from build123d import *

# Parameters (mm, degrees)
SKETCH_1_W      = 303
SKETCH_1_H      = 10
SKETCH_1_R      = 2.025
EXTRUDE_1_DEPTH = 4
FILLET_1_R      = 2


with BuildPart() as part:
    # 草图1 → 凸台-拉伸1 (new body)
    with BuildSketch(Plane.XY):
        Rectangle(SKETCH_1_W, SKETCH_1_H)
        with Locations((-112, 0)):
            Circle(SKETCH_1_R, mode=Mode.SUBTRACT)
        with Locations((-98, 0)):
            Circle(SKETCH_1_R, mode=Mode.SUBTRACT)
        with Locations((-84, 0)):
            Circle(SKETCH_1_R, mode=Mode.SUBTRACT)
        with Locations((-70, 0)):
            Circle(SKETCH_1_R, mode=Mode.SUBTRACT)
        with Locations((-56, 0)):
            Circle(SKETCH_1_R, mode=Mode.SUBTRACT)
        with Locations((-42, 0)):
            Circle(SKETCH_1_R, mode=Mode.SUBTRACT)
        with Locations((-28, 0)):
            Circle(SKETCH_1_R, mode=Mode.SUBTRACT)
        with Locations((-14, 0)):
            Circle(SKETCH_1_R, mode=Mode.SUBTRACT)
        Circle(SKETCH_1_R, mode=Mode.SUBTRACT)
        with Locations((14, 0)):
            Circle(SKETCH_1_R, mode=Mode.SUBTRACT)
        with Locations((28, 0)):
            Circle(SKETCH_1_R, mode=Mode.SUBTRACT)
        with Locations((42, 0)):
            Circle(SKETCH_1_R, mode=Mode.SUBTRACT)
        with Locations((56, 0)):
            Circle(SKETCH_1_R, mode=Mode.SUBTRACT)
        with Locations((70, 0)):
            Circle(SKETCH_1_R, mode=Mode.SUBTRACT)
        with Locations((84, 0)):
            Circle(SKETCH_1_R, mode=Mode.SUBTRACT)
        with Locations((98, 0)):
            Circle(SKETCH_1_R, mode=Mode.SUBTRACT)
        with Locations((112, 0)):
            Circle(SKETCH_1_R, mode=Mode.SUBTRACT)
        with Locations((-144.5, 0)):
            Circle(SKETCH_1_R, mode=Mode.SUBTRACT)
        with Locations((-130.5, 0)):
            Circle(SKETCH_1_R, mode=Mode.SUBTRACT)
        with Locations((130.5, 0)):
            Circle(SKETCH_1_R, mode=Mode.SUBTRACT)
        with Locations((144.5, 0)):
            Circle(SKETCH_1_R, mode=Mode.SUBTRACT)
    extrude(amount=EXTRUDE_1_DEPTH)

    # 圆角1
    fillet_1_edges = [part.edges().sort_by_distance(p)[0] for p in [
        (151.5, -5, 2),
        (-151.5, -5, 2),
        (-151.5, 5, 2),
        (151.5, 5, 2),
    ]]
    fillet(fillet_1_edges, radius=FILLET_1_R)


solid = part.part
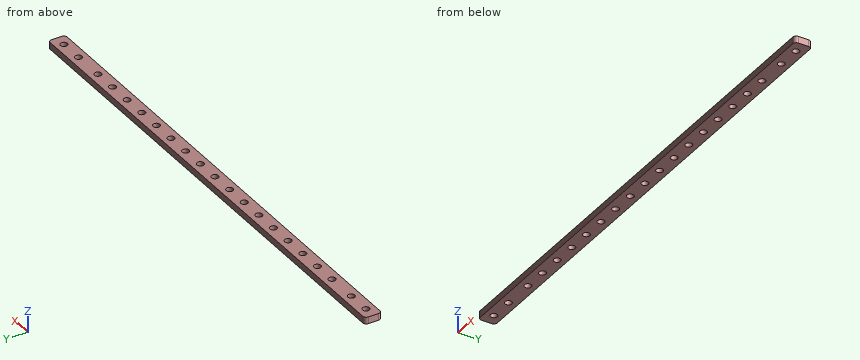
Geometry: final body of the model. Coordinates: model frame, mm. Coordinates: 2 decimals unless noted, no trailing zeros.
(1) First-contact query: pin 1 (4 mm diameter, centred on x = 55, y = 0, fed in from -Z); pin 2 (3 mm diameter, centred on x = -98, y = 0, fed in from -Z). Flat tips, straight axial feed; report the tip coordinate or a pass-through.
(2) Section query A-A (z = 3.2). State how many separate pieces and enclosed holes the cut face has, plus the area to 3 significant figures.
(3) Material intervals for probe 1 along Y at (x, z) = (-14, 0.95) (3 decimals); probe 2 along X at (y, z) = (-3.25, 3.3); probe 3 along Y at (x, z) = (-29, 3.15), sorted ascending.
Solution:
1. pin 1: stops at z = 0
1. pin 2: passes through
2. separate pieces: 1
2. enclosed holes: 21
2. area: 2,760 mm2
3. probe 1: y = -5 to -2.025, 2.025 to 5
3. probe 2: x = -151.48 to 151.48
3. probe 3: y = -5 to -1.76, 1.76 to 5
